```python
from build123d import *

# Parameters (mm, degrees)
F1_DEPTH = 78
F2_R     = 5


# Not quite as in the source:
# - a feature of the source that left no trace in its solid (it failed there, or was rolled back) is left out


with BuildPart() as f1:
    # F0 (on Front) → F1 (new body)
    with BuildSketch(Plane.XZ):
        with BuildLine():
            ThreePointArc((-30.75, -14.9812382666), (-26.6913543678, -16.0682388848), (-23.4375, -18.7265478332))
            ThreePointArc((-23.4375, -18.7265478332), (30, 0), (-23.4375, 18.7265478332))
            ThreePointArc((-23.4375, 18.7265478332), (-26.6913543678, 16.0682388848), (-30.75, 14.9812382666))
            ThreePointArc((-30.75, 14.9812382666), (-45, 0), (-30.75, -14.9812382666))
        make_face()
    extrude(amount=-F1_DEPTH)

    # F2
    f2_edges = [f1.edges().sort_by_distance(p)[0] for p in [
        (30, 0, 0),
        (-26.691354, 0, 16.068239),
        (-45, 0, 0),
        (-26.691354, 0, -16.068239),
    ]]
    fillet(f2_edges, radius=F2_R)


solid = f1.part
```
The listing builds one solid part. Answer for the finished solid, in the listing's coordinates (mm). Round coordinates to 2 decimals unless told otherwise and drop trailing zeros. Loops run counter-clockwise (first coordinate to the right, second up) from the corner with the lowest first, then second, coordinate; pieces in that order, holes last.
1) Given P1, Ø12, axis at y = 59, z = 3.5, coming from the +X side; P2, Ø6, axis at y = 34, z = -4.5, coming from the -X side; P3, Ø2, axis at y = 9.5, z = 20, coming from the -X side, each flat-ended and moving along its own axis, determine where each tip first touches the part or whether it passes through.
Outcome:
P1: stops at x = 30
P2: stops at x = -44.92
P3: stops at x = -23.22
2) A cutting plane is placed at A-A on y = 64. Determine the outline of the cut face in (x, z).
Outcome:
outline: (-30.75, -14.98) arc R10 cw to (-23.44, -18.73) arc R30 ccw (long way) to (-23.44, 18.73) arc R10 cw to (-30.75, 14.98) arc R15 ccw to start
3) Consider line 1 (Y direction, x = -40, z = -2); line 2 (Z direction, x = 20.5, y = 48); line 3 (Z direction, x = 1, y = 33.5). Determine where each line is inside the solid, lowest interval first.
Outcome:
line 1: y = 0 to 78
line 2: z = -21.9 to 21.9
line 3: z = -29.98 to 29.98
